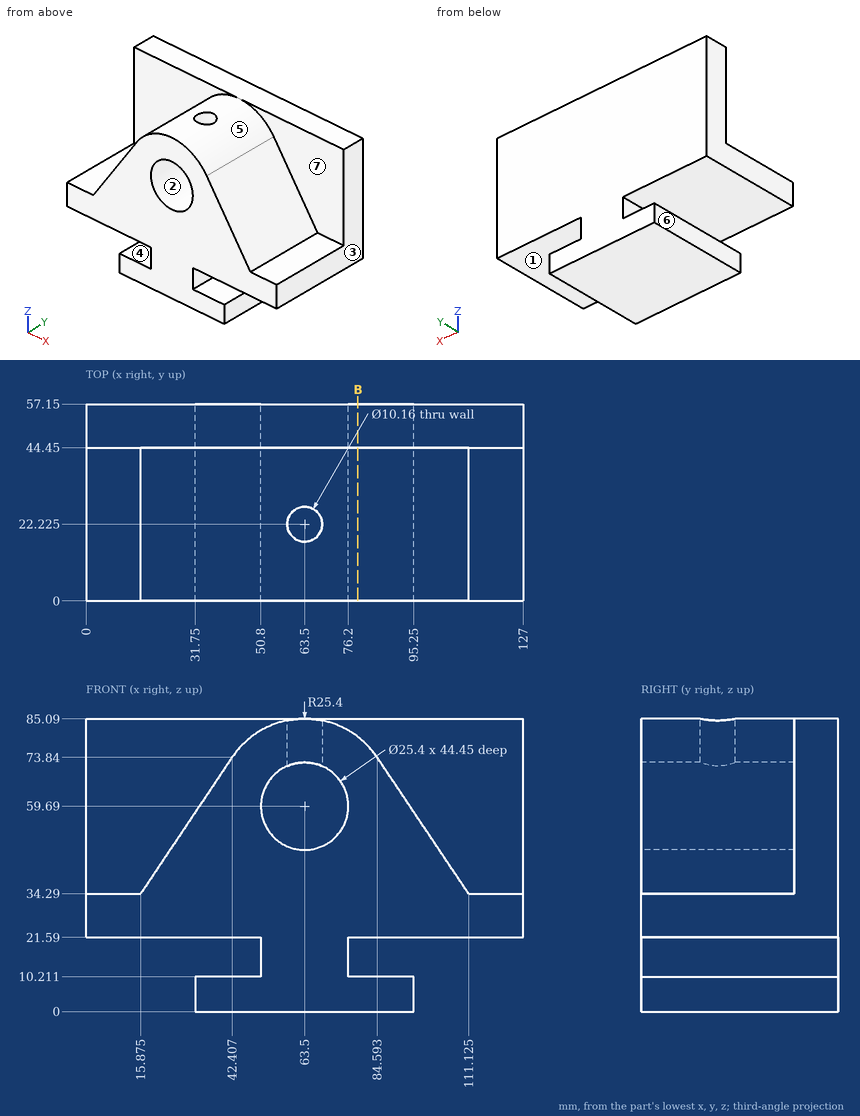
Here's the drawing with two shaded views (mm, measured from the low corner). I have some questions. A direction names the side the tool comes from. Round coordinates to 2 decimals unless told otherwise and drop trailing zeros. Loops run counter-clockwise (first coordinate to the right, second up) from the corner with the lowest first, then second, coordinate; pieces in that order, holes last. Notation, with made-up numbers: M 10.5,20.25 L 57.5,20.25 A22 ccw 57.5,46.25 Z; hole C 33.25,86 d8. An arc over 180 degrees is marked long. Answer as a JSON object with one key per item and string values. Group by question number.
Q1. Will these pins go through, and if not, where does the flat tip stop? pin 1 (2 mm diameter, centred on y = 24, z = 56.5, fed in from -X); pin 2 (3.5 mm diameter, centred on y = 23.5, z = 18, fed in from -X); pin 3 (12.5 mm diameter, centred on x = 11, y = 21, fed in from +Z).
Q2. On a 3-axis mill with a long thin cutter (end or side, diameter ignored), from which of +Z, -Z, +X, -X, +Y, -Y can I reach the whole of each face in a straight line? I mean the marked faces 4, 5, 6 and 7. Say none if no direction works.
Q3. Please list where these lines run through material, in increasing order: L1, parallel to Z at x = 63.5, y = 33; L2, parallel to X at y = 27.5, z = 65 (1 decimal); L3, parallel to Z at x = 86, y = 54.
Q4. We'd pull the mould along X, two halves only. Please class the marked faces 1, 2 and 3: +X half, -X half, draft (parallel to the pull), parting line (faces both ways), or undercut.
Q5. Imagine slicing it at B-B, the plane x = 79. Please give me the cut outline in (y, z), then the cut area to 3 significant figures.
Findings:
{
 "1": {"pin 1": "stops at x = 30.1", "pin 2": "stops at x = 50.8", "pin 3": "stops at z = 36.34"},
 "2": {"face 4": "-X, +Y, -Y", "face 5": "+Z, -Y", "face 6": "-Z, -X, +Y, -Y", "face 7": "+Z, +X, -Y"},
 "3": {"L1": "z = 0 to 46.99, 72.39 to 85.09", "L2": "x = 36.5 to 52, 75 to 90.5", "L3": "z = 0 to 10.21, 21.59 to 85.09"},
 "4": {"face 1": "draft", "face 2": "undercut", "face 3": "+X half"},
 "5": {"outline": "M 0,0 L 57.15,0 L 57.15,10.21 L 0,10.21 Z; M 0,21.59 L 57.15,21.59 L 57.15,85.09 L 44.45,85.09 L 44.45,79.81 L 0,79.81 Z", "area": "3,980 mm2"}
}
